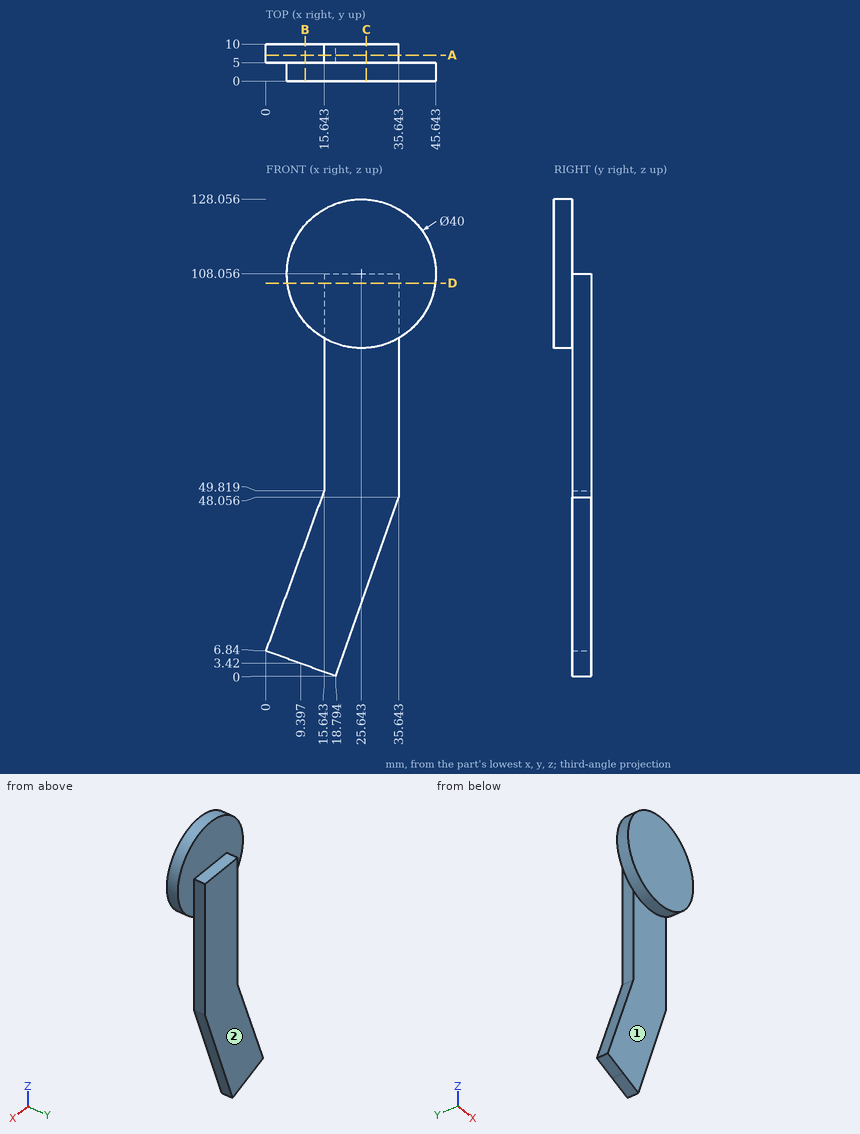
The drawing under review shows one solid part. Ordinate dimensions are in mm from its lowest x, y, z. Round coordinates to 2 decimals unless told otherwise and drop trailing zeros. Loops run counter-clockwise (first coordinate to the right, second up) from the corner with the lowest first, then second, coordinate; pieces in that order, holes last. Notation, with made-up numbers: (-32, -10.75) -> (-26, -10.75) arc R19 cw to (-26, -1.75) -> close; hole circle Ø7 at (23, -32). An arc over 180 degrees is marked (long way). One line per question, with ' | ' between items. Start each with the question number.
Item 1: Wall thickness on line 1 along Y through (x, z) = (12.5, 21.5); line 2 along X through (y, z) = (7, 88); line 3 along Y through (x, z) = (31, 117): over which ranges is each line inside the solid? List them lowest first. Write a range as [from, to].
Item 2: Add section B-B, the plane x = 10.5. Write out the cut boundary in (y, z).
Item 3: Add section C-C, the plane x = 27. Write out the cut boundary in (y, z) (1 decimal), then the cut area to 3 significant figures.
Item 4: For pin 1 (5.5 mm diameter, centred on y = 7, z = 88.5, fed in from +X); pin 2 (5 mm diameter, centred on y = 6.5, z = 100.5, fed in from +X) (1 decimal); pin 3 (6 mm diameter, centred on x = 19.5, y = 6, fed in from +Z), all flat-tipped, find the tip position at first contact; note any pin that passes through.
Item 5: Draft analysis for pull direction Y (two halves, no side actions). For the marked faces 1 and 2, state which applies: +Y half, -Y half, draft (parallel to the pull), parting line (faces both ways), or undercut.
Item 6: Add section A-A, the plane y = 7. Write out the cut boundary in (x, z) (1 decimal).
Item 7: Add section D-D, the plane z = 105.5. Write out the cut boundary in (x, y).
Return value:
1) line 1: y = [5, 10] | line 2: x = [15.64, 35.64] | line 3: y = [0, 5]
2) outline: (0, 94.99) -> (5, 94.99) -> (5, 121.12) -> (0, 121.12) -> close; (5, 3.02) -> (10, 3.02) -> (10, 35.69) -> (5, 35.69) -> close
3) outline: (0, 88.1) -> (5, 88.1) -> (5, 23.4) -> (10, 23.4) -> (10, 108.1) -> (5, 108.1) -> (5, 128) -> (0, 128) -> close | area: 623 mm2
4) pin 1: stops at x = 35.64 | pin 2: stops at x = 44.9 | pin 3: stops at z = 127.78
5) face 1: -Y half | face 2: +Y half
6) outline: (0, 6.8) -> (9.4, 3.4) -> (18.8, 0) -> (35.6, 48.1) -> (35.6, 108.1) -> (15.6, 108.1) -> (15.6, 49.8) -> close
7) outline: (5.81, 0) -> (45.48, 0) -> (45.48, 5) -> (35.64, 5) -> (35.64, 10) -> (15.64, 10) -> (15.64, 5) -> (5.81, 5) -> close
